```python
from build123d import *

# Parameters (mm, degrees)
FILLET_1_R = 0.1


with BuildPart() as part:
    # 草图1 → 旋转1 (revolve)
    with BuildSketch(Plane.XY, mode=Mode.PRIVATE) as revolve_1_sk:
        Polygon((-0.9, 2.4), (-3.578460969, 2.4), (-1.5, 1.2), (-1.5, -4.6), (0, -4.6), (0, 0), (-0.9, 0), align=None)
    revolve(revolve_1_sk.sketch.rotate(Axis((0, -4.6, 0), (0, 1, 0)), 180), axis=Axis((0, -4.6, 0), (0, 1, 0)))

    # 圆角1
    fillet_1_edges = [part.edges().sort_by_distance(p)[0] for p in [
        (-0.9, 0, 0),
        (-1.5, -4.6, 0),
        (-3.578460969, 2.4, 0),
        (-0.9, 2.4, 0),
    ]]
    fillet(fillet_1_edges, radius=FILLET_1_R)


solid = part.part
```
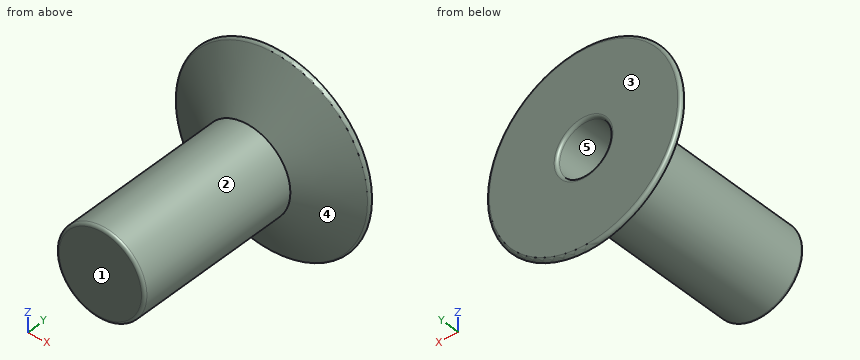
Part model, mm, in its own coordinate system. Face numbers are marked on the shaded views. A direction names the side the tool comes from. Round coordinates to 2 decimals unless told otherwise and drop trailing zeros. Write each loop counter-clockwise with the first axis right and the second up, starting at its lowest first coordinate (ties: lowest second). Pieces come first, ordered by that corner, then holes. Notation, with made-up numbers: (-1.75, -23.75) -> (19.25, -23.75) arc R26 cw to (19.25, 7.25) -> close; hole circle Ø8 at (32.5, -0.5). An arc over 180 degrees is marked (long way). Return JSON: item names as keys, results as strings. Group by question number.
Q1. Saw through at C-C on x = 0. Write the cut outline in (y, z).
Q2. Saw through at B-B on y = 1. Write the cut outline in (x, z).
Q3. Mould opens along X. For the marked faces 3, 4 and 5 say: pulls with the +X half, pulls with the -X half, needs draft (parallel to the pull), parting line crosses it, or undercut.
Q4. Which spindle directions (+Z, -Z, +X, -X, +Y, -Y) get a long thin tool onto all of the face, cutting with end or side? Do the marked faces 1 and 2. Say none if no direction does.
Q5. Saw through at D-D on y = -1.25. Write the cut outline in (x, z).
Q6. Saw through at A-A on z = 0. Write the cut outline in (x, y).
Q7. Pin check, flat tips, straight feed: pin 1 (3 mm diameter, centred on x = -1.5, y = -0.5, fed in from +Z); pin 2 (1.5 mm diameter, centred on y = -3, z = -2.5, fed in from +X); pin 3 (1.6 mm diameter, centred on x = 0, z = 0, fed in from +Y). Stop position of each tip, or through.
Q8. Probe L1, parallel to Z at x = 0, y = 1.1; L2, parallel to Z at x = -0.5, y = 1.75; L3, parallel to X at y = -2.75, z = -0.5. List the from-to ranges inside material, lowest first. Write a range as [from, to].
Answer:
{
 "1": {"outline": "(-4.6, -1.4) arc R0.1 ccw to (-4.5, -1.5) -> (1.2, -1.5) -> (2.21, -3.26) arc R0.1 ccw to (2.4, -3.21) -> (2.4, -1) arc R0.1 ccw to (2.3, -0.9) -> (0.1, -0.9) arc R0.1 cw to (0, -0.8) -> (0, 0.8) arc R0.1 cw to (0.1, 0.9) -> (2.3, 0.9) arc R0.1 ccw to (2.4, 1) -> (2.4, 3.21) arc R0.1 ccw to (2.21, 3.26) -> (1.2, 1.5) -> (-4.5, 1.5) arc R0.1 ccw to (-4.6, 1.4) -> close"},
 "2": {"outline": "circle Ø3 at (0, 0); hole circle Ø1.8 at (0, 0)"},
 "3": {"face 3": "needs draft", "face 4": "parting line crosses it", "face 5": "undercut"},
 "4": {"face 1": "+Z, -Z, +X, -X, -Y", "face 2": "-Y"},
 "5": {"outline": "circle Ø3 at (0, 0)"},
 "6": {"outline": "(-3.26, 2.21) -> (-1.5, 1.2) -> (-1.5, -4.5) arc R0.1 ccw to (-1.4, -4.6) -> (1.4, -4.6) arc R0.1 ccw to (1.5, -4.5) -> (1.5, 1.2) -> (3.26, 2.21) arc R0.1 ccw to (3.21, 2.4) -> (1, 2.4) arc R0.1 ccw to (0.9, 2.3) -> (0.9, 0.1) arc R0.1 cw to (0.8, 0) -> (-0.8, 0) arc R0.1 cw to (-0.9, 0.1) -> (-0.9, 2.3) arc R0.1 ccw to (-1, 2.4) -> (-3.21, 2.4) arc R0.1 ccw to start"},
 "7": {"pin 1": "z = 1.5", "pin 2": "through", "pin 3": "y = 0"},
 "8": {"L1": "[-1.5, -0.9], [0.9, 1.5]", "L2": "[-2.4, -0.75], [0.75, 2.4]", "L3": "[-1.41, 1.41]"}
}
